```python
from build123d import *

# Parameters (mm, degrees)
SKETCH_1_W      = 80
SKETCH_1_H      = 95
SKETCH_1_R      = 7.6
SKETCH_1_R_2    = 2
SKETCH_1_R_3    = 13.2
EXTRUDE_1_DEPTH = 5
FILLET_1_R      = 3


with BuildPart() as part:
    # ｽｹｯﾁ1 → ﾎﾞｽ - 押し出し1 (new body)
    with BuildSketch(Plane(origin=(0, 0, 0), x_dir=(0, 0, -1), z_dir=(1, 0, 0))):
        Rectangle(SKETCH_1_W, SKETCH_1_H)
        with Locations((0, 32.5)):
            Circle(SKETCH_1_R, mode=Mode.SUBTRACT)
        with Locations((12.374368671, -15.125631329)):
            Circle(SKETCH_1_R_2, mode=Mode.SUBTRACT)
        with Locations(Location((12.374368671, -39.874368671, 0), (0, 0, 180))):
            Circle(SKETCH_1_R_2, mode=Mode.SUBTRACT)
        with Locations((-12.374368671, -39.874368671)):
            Circle(SKETCH_1_R_2, mode=Mode.SUBTRACT)
        with Locations(Location((-12.374368671, -15.125631329, 0), (0, 0, 180))):
            Circle(SKETCH_1_R_2, mode=Mode.SUBTRACT)
        with Locations((0, -27.5)):
            Circle(SKETCH_1_R_3, mode=Mode.SUBTRACT)
        with Locations((32.5, 40)):
            Circle(SKETCH_1_R_2, mode=Mode.SUBTRACT)
        with Locations(Location((32.5, -40, 0), (0, 0, 180))):
            Circle(SKETCH_1_R_2, mode=Mode.SUBTRACT)
        with Locations((-32.5, -40)):
            Circle(SKETCH_1_R_2, mode=Mode.SUBTRACT)
        with Locations(Location((-32.5, 40, 0), (0, 0, 180))):
            Circle(SKETCH_1_R_2, mode=Mode.SUBTRACT)
    extrude(amount=EXTRUDE_1_DEPTH)

    # ﾌｨﾚｯﾄ1
    fillet_1_edges = [part.edges().sort_by_distance(p)[0] for p in [
        (2.5, -47.5, -40),
        (2.5, -47.5, 40),
        (2.5, 47.5, 40),
        (2.5, 47.5, -40),
    ]]
    fillet(fillet_1_edges, radius=FILLET_1_R)


solid = part.part
```
Design review of the part built by this model. Coordinates are the model's own, in mm. Give positions to 0.01 mm unless a question says otherwise; leave off trailing zeros. Order: outer loops, then holes, each group sorted by start corner. A loop starts at its lowest first (then second) coordinate and runs counter-clockwise, first axis right, second up. Notation, with made-up numbers: (5.5, 42.5) -> (27.5, 42.5) arc R28 ccw to (27.5, 72.5) -> close; hole circle Ø7 at (16, 45). An arc over 180 degrees is marked (long way). Write item = value, one per line. Start each with the question number.
(1) We need section A-A on z = 32.5. Write out the cut boundary in (x, y), plus the area to 3 significant figures.
(2) Mouldability with a two-part tool opening along Y and no side actions: class faces 1 (the face through (2, -47.5, 1)), 2 (the face through (2.465, -38.226, -31.577)), 3 (the face through (2.465, 38.226, -33.423)), 4 (the face through (2.54, 46.6, 39.14)) as +Y half, -Y half, draft (parallel to the pull), parting line (faces both ways), or undercut.
(3) To check wall thickness, follow line 1 along Y through (x, z) = (1.15, -32.5); line 2 along Y through (x, z) = (0.75, 33); line 3 along Z through (x, y) = (1.55, 33). State the ranges of each line that lie inside material, in increasing order.
(4) We need section C-C on z = 0. Write out the cut boundary in (x, y).
(5) We need section D-D on x = 3. State how many separate pieces and enclosed holes the cut face has, plus the area to 3 significant figures.
(6) For pin 1 (3 mm diameter, centred on y = 40, z = -32.5, fed in from -X), flat-tipped, find the tip position at first contact; note if it passes through.
(7) We need section B-B on y = -36.5. Write out the cut boundary in (x, z).
Numbers:
q1.outline = (0, -47.5) -> (5, -47.5) -> (5, -42) -> (0, -42) -> close; (0, -38) -> (5, -38) -> (5, 38) -> (0, 38) -> close; (0, 42) -> (5, 42) -> (5, 47.5) -> (0, 47.5) -> close
q1.area = 435 mm^2
q2.face_1 = -Y half
q2.face_2 = undercut
q2.face_3 = undercut
q2.face_4 = +Y half
q3.line_1 = -47.5 to -42, -38 to 38, 42 to 47.5
q3.line_2 = -47.5 to -41.94, -38.06 to 38.06, 41.94 to 47.5
q3.line_3 = -40 to -7.58, 7.58 to 40
q4.outline = (0, -47.5) -> (5, -47.5) -> (5, -40.7) -> (0, -40.7) -> close; (0, -14.3) -> (5, -14.3) -> (5, 24.9) -> (0, 24.9) -> close; (0, 40.1) -> (5, 40.1) -> (5, 47.5) -> (0, 47.5) -> close
q5.separate_pieces = 1
q5.enclosed_holes = 10
q5.area = 6,760 mm^2
q6.pin_1 = through
q7.outline = (0, -40) -> (5, -40) -> (5, -9.66) -> (0, -9.66) -> close; (0, 9.66) -> (5, 9.66) -> (5, 40) -> (0, 40) -> close
